from build123d import *

# Parameters (mm, degrees)
SKETCH1_W             = 23
SKETCH1_H             = 21
EXTRUDE1_DEPTH        = 5
SKETCH2_R             = 2.15
EXTRUDE2_DEPTH        = 4.5
SKETCH4_R             = 1.25
EXTRUDE4_DEPTH        = 8
FILLET1_R             = 5
SKETCH6_R             = 4.5
EXTRUDE6_DEPTH        = 4.5
SKETCH9_W             = 12
SKETCH9_H             = 26
EXTRUDE9_DEPTH        = 5
SKETCH11_R            = 1.5
EXTRUDE11_DEPTH       = 5
SKETCH10_R            = 2
EXTRUDE10_DEPTH       = 4
M3_TAPPED_HOLE1_D     = 2.5
M3_TAPPED_HOLE1_DEPTH = 8
M3_TAPPED_HOLE1_TIP   = 0.751075774
EXTRUDE12_DEPTH       = 4
FILLET3_R             = 3
EXTRUDE14_DEPTH       = 4
FILLET4_R             = 2
EXTRUDE15_DEPTH       = 5
FILLET6_R             = 2


with BuildPart() as part:
    # Sketch1 → Extrude1 (new body)
    with BuildSketch(Plane.XY):
        with Locations((3.5, -4)):
            Rectangle(SKETCH1_W, SKETCH1_H)
    extrude(amount=EXTRUDE1_DEPTH)

    # Sketch2 → Extrude2 (cut)
    with BuildSketch(Plane.XY.offset(5)):
        with Locations((6, 0)):
            Circle(SKETCH2_R)
    extrude(amount=-EXTRUDE2_DEPTH, mode=Mode.SUBTRACT)

    # Sketch4 → Extrude4 (cut)
    with BuildSketch(Plane.XZ.offset(14.5)):
        with Locations(Location((-1.4, 2.5, 0), (0, 0, 270))):
            Circle(SKETCH4_R)
        with Locations(Location((12, 2.5, 0), (0, 0, 270))):
            Circle(SKETCH4_R)
    extrude(amount=-EXTRUDE4_DEPTH, mode=Mode.SUBTRACT)

    # Fillet1
    fillet1_edges = [part.edges().sort_by_distance(p)[0] for p in [
        (15, 6.5, 2.5),
    ]]
    fillet(fillet1_edges, radius=FILLET1_R)

    # Sketch6 → Extrude6 (cut)
    with BuildSketch(Plane(origin=(0, 0, 0), x_dir=(-1, 0, 0), z_dir=(0, 0, -1))):
        with Locations((-4.9, -6.5)):
            Circle(SKETCH6_R)
    extrude(amount=-EXTRUDE6_DEPTH, mode=Mode.SUBTRACT)

    # Sketch9 → Extrude9 (add)
    with BuildSketch(Plane(origin=(0, 0, 0), x_dir=(-1, 0, 0), z_dir=(0, 0, -1))):
        with Locations((14, -6.5)):
            Rectangle(SKETCH9_W, SKETCH9_H)
    extrude(amount=-EXTRUDE9_DEPTH)

    # Sketch11 → Extrude11 (cut)
    with BuildSketch(Plane.XY.offset(5)):
        with Locations((-17.5, -5.5)):
            Circle(SKETCH11_R)
    extrude(amount=-EXTRUDE11_DEPTH, mode=Mode.SUBTRACT)

    # Sketch10 → Extrude10 (cut)
    with BuildSketch(Plane.XY.offset(5)):
        with Locations((-10, -2.5)):
            Circle(SKETCH10_R)
    extrude(amount=-EXTRUDE10_DEPTH, mode=Mode.SUBTRACT)

    # M3 Tapped Hole1
    with Locations(Plane(origin=(-1.4, -14.5, 2.5), x_dir=(0, 0, -1), z_dir=(0, -1, 0))):
        with Locations((0, 0), (0, 13.4)):
            Hole(M3_TAPPED_HOLE1_D / 2, depth=M3_TAPPED_HOLE1_DEPTH)
            with Locations((0, 0, -(M3_TAPPED_HOLE1_DEPTH + M3_TAPPED_HOLE1_TIP / 2))):  # 118° drill point
                Cone(0, M3_TAPPED_HOLE1_D / 2, M3_TAPPED_HOLE1_TIP, mode=Mode.SUBTRACT)

    # Sketch13 → Extrude12 (add)
    with BuildSketch(Plane(origin=(0, 0, 0), x_dir=(-1, 0, 0), z_dir=(0, 0, -1))):
        Polygon((20, -19.5), (8, -19.5), (8, -14.5), (2, -14.5), (2, -11.07), (18.1, 1), (20, 1), align=None)
    extrude(amount=EXTRUDE12_DEPTH)

    # Fillet3
    fillet3_edges = [part.edges().sort_by_distance(p)[0] for p in [
        (-20, -19.5, 0.5),
        (-20, 6.5, 2.5),
    ]]
    fillet(fillet3_edges, radius=FILLET3_R)

    # Sketch14 → Extrude14 (cut)
    with BuildSketch(Plane(origin=(0, 0, -4), x_dir=(-1, 0, 0), z_dir=(0, 0, -1))):
        Polygon((19.5, 1), (19.5, -7.5), (15.5, -7.5), (15.5, -0.949192547), (18.1, 1), align=None)
    extrude(amount=-EXTRUDE14_DEPTH, mode=Mode.SUBTRACT)

    # Fillet4
    fillet4_edges = [part.edges().sort_by_distance(p)[0] for p in [
        (-19.5, -7.5, -2),
        (-15.5, -7.5, -2),
    ]]
    fillet(fillet4_edges, radius=FILLET4_R - 0.0001)  # a hair under: the kernel refuses the full size

    # Sketch15 → Extrude15 (cut)
    with BuildSketch(Plane.XY.offset(5)):
        Polygon((-14, 2.5), (-17, 6.5), (-7, 6.5), (-10, 2.5), align=None)
    extrude(amount=-EXTRUDE15_DEPTH, mode=Mode.SUBTRACT)

    # Fillet6
    fillet6_edges = [part.edges().sort_by_distance(p)[0] for p in [
        (-10, 2.5, 2.5),
        (-14, 2.5, 2.5),
    ]]
    fillet(fillet6_edges, radius=FILLET6_R)


solid = part.part
Can you work these out from the model? Positions are in its coordinate system, mm. A direction names the side the tool comes from. Coordinates: 2 decimals unless noted, no trailing zeros. Write each loop counter-clockwise with the first axis right and the second up, starting at its lowest first coordinate (ties: lowest second). Pieces come first, ordered by that corner, then holes. Notation, with made-up numbers: (-4.75, 11.25) -> (37.25, 11.25) arc R20 cw to (37.25, 23.25) -> close; hole circle Ø6 at (35, -7). An arc over 180 degrees is marked (long way). Write each question's results on one line, items separated by ' | '. Start each with the question number.
Item 1: Please list where these lines run through material, in increasing order: probe 1 along X at (y, z) = (-11.25, 2.5); probe 2 along Z at (x, y) = (12, -12.25); probe 3 along X at (y, z) = (0, 2.35).
Item 2: If we section it at B-B, the plane x = -18: Write out the boundary of the cut face in (y, z), and give its area (3 significant figures).
Item 3: If we section it at A-A, the plane y = -12.5: Write out the boundary of the cut face in (x, z).
Item 4: On a 3-axis mill with a long thin cutter (end or side, diameter ignored), from which of +Z, -Z, +X, -X, +Y, -Y can I reach the whole of each face in a straight line? I mean faces 1 (the cylindrical face through (13.054, -10.556, 1.828)), 2 (the flat face through (-19.5, -2, -2)), 3 (the flat face through (-12, 2.5, 3)), 4 (the flat face through (5, -6, 4.5)), 5 (the cylindrical face through (5.72, 2.13, 2.78)). Say none if no direction works.
Item 5: If we section it at D-D, the plane y = -3.25: Write out the boundary of the cut face in (x, z), and give its area (3 significant figures).
Item 6: Thinking about a two-plate mould opening in X: for faces 6 (the flat face through (-8, -17, 1)), 7 (the flat face through (-20, -6, 1)), 8 (the flat face through (1, -14.5, 2)), 9 (the cylindrical face through (2.82, -10.49, 2.22)), which applies, released by +X, released by -X, zero draft, split by the parting line, or undercut?
Item 7: I'm going to push flat-ended pins straight in: P1, Ø3, axis at y = 2, z = -1.5, coming from the -X side; P2, Ø1.7, axis at y = -13, z = -2, coming from the +X side; P3, Ø1.5, axis at x = 6.5, y = -7.5, coming from the -Z side; P4, Ø2, axis at x = 12, z = 2.5, coming from the -Y side. Where does each tip first touch, or does it pass through?
Answer block:
1) probe 1: -20 to -2.65, -0.15 to 10.75, 13.25 to 15 | probe 2: 0 to 1.25, 3.75 to 5 | probe 3: -20 to 3.85, 8.15 to 15
2) outline: (-19.33, -4) -> (-7.44, -4) -> (-7.44, 0) -> (-6.91, 0) -> (-6.91, 5) -> (-19.33, 5) -> close; (-4.09, 0) -> (6.33, 0) -> (6.33, 5) -> (-4.09, 5) -> close | area: 162 mm²
3) outline: (-20, -4) -> (-2, -4) -> (-2, 0) -> (15, 0) -> (15, 5) -> (-20, 5) -> close; hole circle Ø2.5 at (-1.4, 2.5); hole circle Ø2.5 at (12, 2.5)
4) face 1: -Y | face 2: -Z, +Y | face 3: +Z, -Z, +Y | face 4: -Z | face 5: +Z
5) outline: (-20, -4) -> (-19.5, -4) -> (-19.5, 0) -> (-15.5, 0) -> (-15.5, -4) -> (-12.43, -4) -> (-12.43, 0) -> (1.79, 0) -> (1.79, 4.5) -> (8.01, 4.5) -> (8.01, 0) -> (15, 0) -> (15, 5) -> (-8.15, 5) -> (-8.15, 1) -> (-11.85, 1) -> (-11.85, 5) -> (-20, 5) -> close | area: 146 mm²
6) face 6: released by +X | face 7: released by -X | face 8: zero draft | face 9: undercut
7) P1: x = -20 | P2: x = -2 | P3: z = 4.5 | P4: y = -6.35
